from build123d import *

# Parameters (mm, degrees)
SKETCH3_R          = 3.175
CUT_EXTRUDE1_DEPTH = 10


with BuildPart() as part:
    # Sketch1 → Revolve1 (revolve)
    with BuildSketch(Plane.XY):
        Polygon((83, 5), (70, 5), (70, 20), (60, 20), (60, 5), (10, 5), (10, 23.975), (0, 23.975), (0, 0), (83, 0), align=None)
    revolve(axis=Axis((0, 0, 0), (1, 0, 0)))

    # Sketch3 → Cut-Extrude1 (cut)
    with BuildSketch(Plane.ZY):
        with Locations((0, 19.05)):
            Circle(SKETCH3_R)
        with Locations((19.05, 0)):
            Circle(SKETCH3_R)
        with Locations((0, -19.05)):
            Circle(SKETCH3_R)
        with Locations((-19.05, 0)):
            Circle(SKETCH3_R)
    extrude(amount=-CUT_EXTRUDE1_DEPTH, mode=Mode.SUBTRACT)


solid = part.part
The listing builds one solid part. Answer for the finished solid, in the listing's coordinates (mm). A direction names the side the tool comes from. Coordinates: 2 decimals unless noted, no trailing zeros. Order: outer loops, then holes, each group sorted by start corner. A loop starts at its lowest first (then second) coordinate and runs counter-clockwise, first axis right, second up.
Q1. Which of the six approach directions +Z, -Z, +X, -X, +Y, -Y give full straight-line access (tool end or side, diameter ignored) to faces 4 (the face through (4.93, -17.671, 16.203)), 5 (the face through (70, -4, -4)), 6 (the face through (4.93, 15.95, -0.69)), 7 (the face through (34.65, -1.08, -4.88))?
Q2. A cutting plane is placed at C-C, the plane x = 9. Write down the section's boundary in (y, z) (3 decimals), and give its area (3 significant figures).
Q3. A cutting plane is placed at A-A, the plane z = 0. Write down the section's boundary in (x, y) (3 decimals).
Q4. A cutting plane is placed at D-D, the plane y = 15. Write down the section's boundary in (x, z), and give its area (3 significant figures).
Q5. For a pull along X with two mould halves and no side action, classify faces 1 (the face through (60, 4, -4)), 2 (the face through (0, 0, 0)), 3 (the face through (76.41, -1.08, -4.88)) as pulls with the +X half, pulls with the -X half, needs draft (parallel to the pull), parting line crosses it, or undercut.
Q6. Consider line 1 (X direction, y = 17, z = 8); line 2 (X direction, y = 18.5, z = -8.5); line 3 (Y direction, x = 21, z = 4.5). Determine where each line is inside the solid, lowest interval first.
Q7. Given P1, Ø10, axis at x = 10.5, y = -5, coming from the +Z side (3 decimals); P2, Ø6, axis at x = 58.5, y = -8, coming from the -Z side; P3, Ø2, axis at x = 66.5, z = -4, coming from the +Y side, each flat-ended and moving along its own axis, determine where each tip first touches the part or whether it passes through.
Answers follow:
1. face 4: +X, -X
1. face 5: +X
1. face 6: -X
1. face 7: none
2. outline: circle Ø47.95 at (0, 0); hole circle Ø6.35 at (-19.05, 0); hole circle Ø6.35 at (0, -19.05); hole circle Ø6.35 at (0, 19.05); hole circle Ø6.35 at (19.05, 0)
2. area: 1,680 mm2
3. outline: (0, -23.975) - (10, -23.975) - (10, -22.225) - (0, -22.225) - close; (0, -15.875) - (10, -15.875) - (10, -5) - (60, -5) - (60, -20) - (70, -20) - (70, -5) - (83, -5) - (83, 5) - (70, 5) - (70, 20) - (60, 20) - (60, 5) - (10, 5) - (10, 15.875) - (0, 15.875) - close; (0, 22.225) - (10, 22.225) - (10, 23.975) - (0, 23.975) - close
4. outline: (0, -18.7) - (10, -18.7) - (10, 18.7) - (0, 18.7) - close; (60, -13.23) - (70, -13.23) - (70, 13.23) - (60, 13.23) - close
4. area: 639 mm2
5. face 1: undercut
5. face 2: pulls with the -X half
5. face 3: needs draft
6. line 1: x = 0 to 10, 60 to 70
6. line 2: x = 0 to 10
6. line 3: y = -2.18 to 2.18
7. P1: stops at z = 23.975
7. P2: stops at z = -19.26
7. P3: stops at y = 19.77
